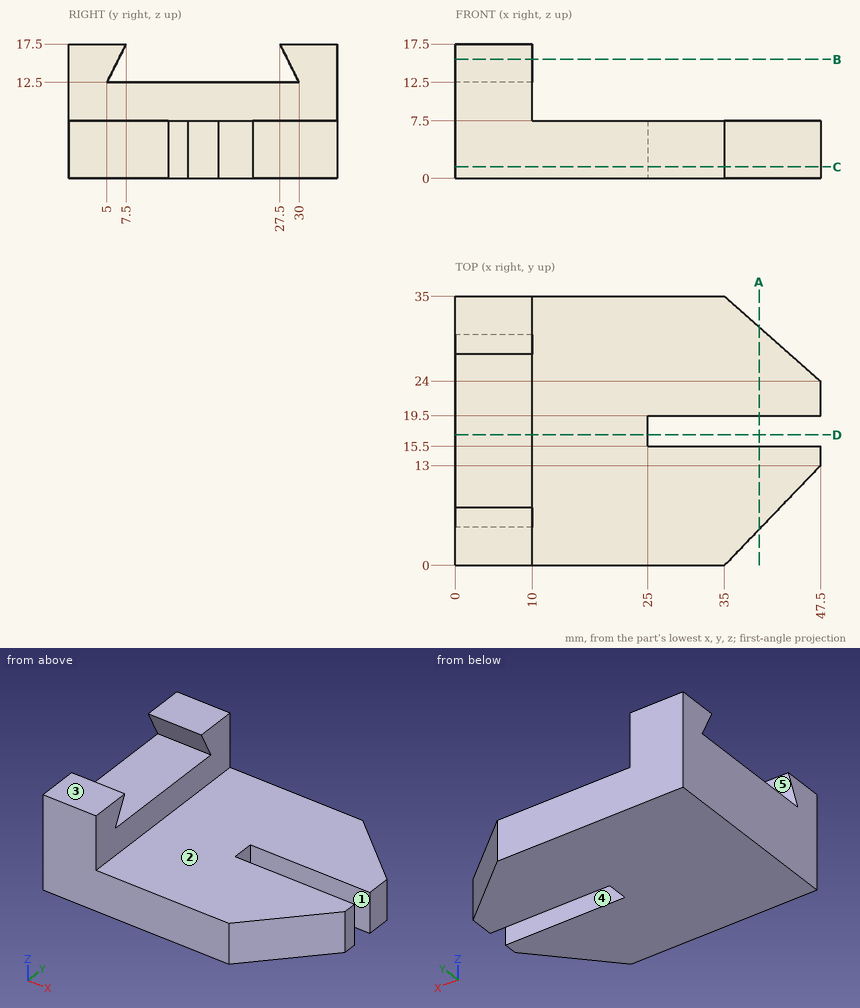
Geometry check sheet. Reference: drawing and pictorial views, mm from the part's lowest x, y, z. A direction names the side the tool comes from. Round coordinates to 2 decimals unless told otherwise and drop trailing zeros. Loops run counter-clockwise (first coordinate to the right, second up) from the corner with the lowest first, then second, coordinate; pieces in that order, holes last. Notation, with made-up numbers: (-38, 58) -> (-10, 58) arc R29 ccw to (-10, 91) -> close; hole circle Ø11 at (79.25, 46.5). An arc over 180 degrees is marked (long way). Answer as a JSON object with one key per item and string values. Group by question number.
Item 1: Cross-section at B-B, the plane z = 15.5. Record the cut outline in (x, y), plus the area to 3 significant figures.
Item 2: Set-up check for the marked faces 1 and 2: record each of +Z, -Z, +X, -X, +Y, -Y from which the full face is reachable in a straight line by a thin tool's end or side.
Item 3: Depth check by flat-ended pin: pin 1 Ø6 at (x, z) = (41.5, 4) entering from -Y; pin 2 Ø10.5 at (x, y) = (29.5, 23) entering from +Z; pin 3 Ø3 at (y, z) = (14, 12.5) entering from +X. Enter the tip coordinate at first touch or a pass-through.
Item 4: Cross-section at C-C, the plane z = 1.5. Record the cut outline in (x, y), plus the area to 3 significant figures.
Item 5: Thickness scan on line 1 along Z through (x, y) = (36, 31.5); line 2 along Z through (x, y) = (8, 19); line 3 along X through (y, z) = (16.5, 6.5). Record the ranges inside material, lowest first.
Item 6: Cross-section at A-A, the plane x = 39.5. Record the cut outline in (y, z).
Item 7: Release check for a two-part mould opening along Z. For the marked faces 3, 4 and 5 record: pulls with the +Z half, pulls with the -Z half, needs draft (parallel to the pull), parting line crosses it, or undercut.
Item 8: Cross-section at D-D, the plane y = 17. Record the cut outline in (x, z).
Determined:
{
 "1": {"outline": "(0, 0) -> (10, 0) -> (10, 6.5) -> (0, 6.5) -> close; (0, 28.5) -> (10, 28.5) -> (10, 35) -> (0, 35) -> close", "area": "130 mm²"},
 "2": {"face 1": "+Z, -Z, +X", "face 2": "+Z, +X, +Y, -Y"},
 "3": {"pin 1": "stops at y = 3.64", "pin 2": "stops at z = 7.5", "pin 3": "stops at x = 10"},
 "4": {"outline": "(0, 0) -> (35, 0) -> (47.5, 13) -> (47.5, 15.5) -> (25, 15.5) -> (25, 19.5) -> (47.5, 19.5) -> (47.5, 24) -> (35, 35) -> (0, 35) -> close", "area": "1,420 mm²"},
 "5": {"line 1": "z = 0 to 7.5", "line 2": "z = 0 to 12.5", "line 3": "x = 0 to 25"},
 "6": {"outline": "(4.68, 0) -> (15.5, 0) -> (15.5, 7.5) -> (4.68, 7.5) -> close; (19.5, 0) -> (31.04, 0) -> (31.04, 7.5) -> (19.5, 7.5) -> close"},
 "7": {"face 3": "pulls with the +Z half", "face 4": "needs draft", "face 5": "undercut"},
 "8": {"outline": "(0, 0) -> (25, 0) -> (25, 7.5) -> (10, 7.5) -> (10, 12.5) -> (0, 12.5) -> close"}
}
